The model under review builds one solid part; all positions refer to its coordinate system, in mm. A direction names the side the tool comes from. Give positions to 0.01 mm unless a question says otherwise; leave off trailing zeros. Loops run counter-clockwise (first coordinate to the right, second up) from the corner with the lowest first, then second, coordinate; pieces in that order, holes last. Notation, with made-up numbers: M 10,41 L 40,41 A24 cw 40,74 Z; hole C 37,-38.75 d9. An arc over 180 degrees is marked long. Return JSON: item names as keys, results as strings.
```python
from build123d import *

# Parameters (mm, degrees)
SKETCH1_R           = 5
SKETCH1_R_2         = 2.5
SKETCH1_R_3         = 1.5
BOSS_EXTRUDE1_DEPTH = 6.4
SKETCH2_R           = 3
CUT_EXTRUDE1_DEPTH  = 3
CHAMFER1_SIZE       = 5
FILLET1_R           = 20


with BuildPart() as part:
    # Sketch1 → Boss-Extrude1 (new body)
    with BuildSketch(Plane.XY):
        with BuildLine():
            Line((150, 19.05), (16.189425561, 19.05))
            ThreePointArc((16.189425561, 19.05), (-25, 0), (16.189425561, -19.05))
            Line((16.189425561, -19.05), (150, -19.05))
            Line((150, -19.05), (150, 19.05))
        make_face()
        Circle(SKETCH1_R, mode=Mode.SUBTRACT)
        with Locations((130, 10)):
            Circle(SKETCH1_R_2, mode=Mode.SUBTRACT)
        with Locations((110, 10)):
            Circle(SKETCH1_R_2, mode=Mode.SUBTRACT)
        with Locations((110, -10)):
            Circle(SKETCH1_R_2, mode=Mode.SUBTRACT)
        with Locations((130, -10)):
            Circle(SKETCH1_R_2, mode=Mode.SUBTRACT)
        with Locations((0, 12.7)):
            Circle(SKETCH1_R_3, mode=Mode.SUBTRACT)
        with Locations((0, -12.7)):
            Circle(SKETCH1_R_3, mode=Mode.SUBTRACT)
        with Locations((12.7, 0)):
            Circle(SKETCH1_R_3, mode=Mode.SUBTRACT)
        with Locations((-12.7, 0)):
            Circle(SKETCH1_R_3, mode=Mode.SUBTRACT)
    extrude(amount=BOSS_EXTRUDE1_DEPTH)

    # Sketch2 → Cut-Extrude1 (cut)
    with BuildSketch(Plane.XY.offset(6.4)):
        with Locations((0, 12.7)):
            Circle(SKETCH2_R)
        with Locations((12.7, 0)):
            Circle(SKETCH2_R)
        with Locations((0, -12.7)):
            Circle(SKETCH2_R)
        with Locations((-12.7, 0)):
            Circle(SKETCH2_R)
    extrude(amount=-CUT_EXTRUDE1_DEPTH, mode=Mode.SUBTRACT)

    # Chamfer1
    chamfer1_edges = [part.edges().sort_by_distance(p)[0] for p in [
        (150, -19.05, 3.2),
        (150, 19.05, 3.2),
    ]]
    chamfer(chamfer1_edges, length=CHAMFER1_SIZE)

    # Fillet1
    fillet1_edges = [part.edges().sort_by_distance(p)[0] for p in [
        (16.189425561, -19.05, 3.2),
        (16.189425561, 19.05, 3.2),
    ]]
    fillet(fillet1_edges, radius=FILLET1_R)


solid = part.part
```
1) Wall thickness on L1, parallel to Y at x = 0, z = 4.25; L2, parallel to Y at x = 0, z = 2.1; L3, parallel to Y at x = 110, z = 2.75: over which ranges is each line inside the solid? List them lowest first. Write a range as from..to.
From the geometry:
{"L1": "-25..-15.7, -9.7..-5, 5..9.7, 15.7..25", "L2": "-25..-14.2, -11.2..-5, 5..11.2, 14.2..25", "L3": "-19.05..-12.5, -7.5..7.5, 12.5..19.05"}
2) Insertion check: pin 1 (1 mm diameter, centred on x = 27.5, z = 3, fed in from -Y); pin 2 (3.5 mm diameter, centred on x = 0, y = 12.7, fed in from +Z); pin 3 (2.5 mm diameter, centred on x = 0, y = -12.7, fed in from -Z); pin 4 (2 mm diameter, centred on x = 116.5, z = 1.5, fed in from +Y). Each pin has a flat end and moves straight along its axis. Give the tip position at first contact, or say it passes through.
From the geometry:
{"pin 1": "y = -19.05", "pin 2": "z = 3.4", "pin 3": "through", "pin 4": "y = 19.05"}
3) Consider section C-C on x = -12.7. Write out the cut boundary in (y, z).
From the geometry:
{"outline": "M -21.53,0 L -1.5,0 L -1.5,3.4 L -3,3.4 L -3,6.4 L -21.53,6.4 Z; M 1.5,0 L 21.53,0 L 21.53,6.4 L 3,6.4 L 3,3.4 L 1.5,3.4 Z"}
4) Tool access review of faces 4 (the face through (-0.325, 11.236, 1.676)), 5 (the face through (-0.391, -9.726, 4.921)): name each direction out of +Z, -Z, +X, -X, +Y, -Y from which nothing blocks a thin tool from reaching the whole face with its end or side.
From the geometry:
{"face 4": "+Z, -Z", "face 5": "+Z"}
5) Consider section A-A on x = 110. Write out the cut boundary in (y, z).
From the geometry:
{"outline": "M -19.05,0 L -12.5,0 L -12.5,6.4 L -19.05,6.4 Z; M -7.5,0 L 7.5,0 L 7.5,6.4 L -7.5,6.4 Z; M 12.5,0 L 19.05,0 L 19.05,6.4 L 12.5,6.4 Z"}
6) Consider section B-B on z = 1.75. Count the separate pieces of the cut face and the enclosed holes in it, then the cut area to 3 significant figures.
From the geometry:
{"separate pieces": "1", "enclosed holes": "9", "area": "6,620 mm²"}
7) The part is to be moulded in two halves that separate along Y. For faces 1 (the face through (85, 19.05, 3)), 2 (the face through (11, -1, 3.4)), 3 (the face through (-24.99, 0.73, 3.16)), say which applies: released by +Y, released by -Y, zero draft, split by the parting line, or undercut.
From the geometry:
{"face 1": "released by +Y", "face 2": "undercut", "face 3": "split by the parting line"}
